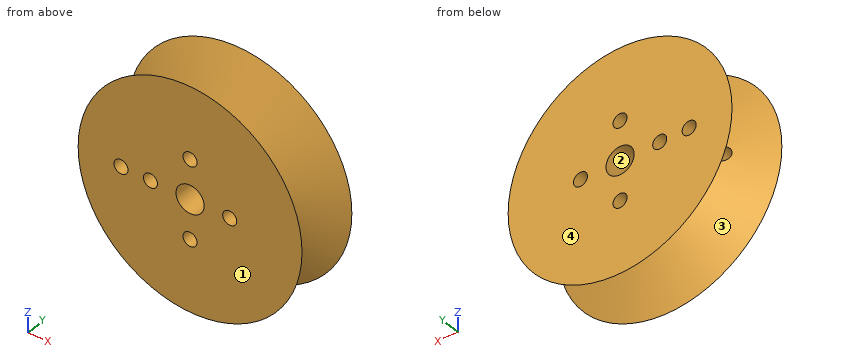
Autodesk Inventor part; units mm, degrees
ref_plane "YZ Plane" through (0, 0, 0) normal (1, 0, 0) x (0, 1, 0)
ref_plane "XZ Plane" through (0, 0, 0) normal (0, 1, 0) x (-1, 0, 0)
ref_plane "XY Plane" through (0, 0, 0) normal (0, 0, 1) x (1, 0, 0)
sketch "Sketch1" plane through (0, 0, 0) normal (0, 1, 0) x (-1, 0, 0)
  circle A0 centre (0, 0) radius 22.225
  dimension "d0" = 44.45
extrude "Extrusion1" add sketch "Sketch1" along normal blind 6.35
chamfer "Chamfer1" distance 12.7 distance2 6.35 1 edges at (22.225, 6.35, 0) measured on face at (-2.0252, 6.35, -4.4852)
sketch "Sketch2" plane through (0, 6.35, 0) normal (0, 1, 0) x (1, 0, 0)
  circle A0 centre (0, 0) radius 22.225
  dimension "d57" = 44.45
extrude "Extrusion2" add sketch "Sketch2" along normal blind 6.35
chamfer "Chamfer2" distance 12.7 distance2 6.35 1 edges at (-22.225, 6.35, 0) measured on face at (17.7764, 6.35, 1.7729)
sketch "Sketch4" plane through (0, 12.7, 0) normal (0, 1, 0) x (1, 0, 0)
  circle A0 centre (0, 0) radius 2.794
  line L0 (0, 0) -> (-7.874, 0)
  line L1 (-7.874, 0) -> (-13.716, 0)
  line L2 (0, 0) -> (0, 7.874)
  line L3 (0, 0) -> (7.874, 0)
  line L4 (0, 0) -> (0, -7.874)
  circle A1 centre (0, -7.874) radius 1.397
  circle A2 centre (7.874, 0) radius 1.397
  circle A3 centre (0, 7.874) radius 1.397
  circle A4 centre (-7.874, 0) radius 1.397
  circle A5 centre (-13.716, 0) radius 1.397
  dimension "d28" = 5.588
  dimension "d29" = 7.874
  dimension "d30" = 5.842
  dimension "d31" = 7.874
  dimension "d32" = 7.874
  dimension "d33" = 7.874
  dimension "d34" = 2.794
  dimension "d35" = 2.794
  dimension "d36" = 2.794
  dimension "d37" = 2.794
  dimension "d38" = 2.794
extrude "Extrusion3" cut sketch "Sketch4" against normal blind 15.24
sketch "Sketch5" plane through (0, 0, 0) normal (0, -1, 0) x (1, 0, 0)
  circle A0 centre (0, 0) radius 2.794
  circle A1 centre (0, 0) radius 11.1125
  dimension "d58" = 22.225
properties part number "String Little Big Wheel V5"
The listing builds one solid part. Answer for the finished solid, in the listing's coordinates (mm). Face numbers are marked on the shaded views. A direction names the side the tool comes from. Coordinates: 2 decimals unless noted, no trailing zeros. Write each loop counter-clockwise with the first axis right and the second up, starting at its lowest first coordinate (ties: lowest second). Pieces come first, ordered by that corner, then holes. Notation, with made-up numbers: (37.25, -11.75) - (84.25, -11.75) arc R33 ccw to (84.25, 23.25) - close; hole circle Ø6 at (-35.75, 57). An arc over 180 degrees is marked (long way). Return JSON: item names as keys, results as strings.
1. Which of the six approach directions +Z, -Z, +X, -X, +Y, -Y give full straight-line access (tool end or side, diameter ignored) to the marked faces 3 and 4?
Final values:
{"face 3": "none", "face 4": "+Z, -Z, +X, -X, +Y"}
2. The part is cut by section A-A on z = 0. Count the separate pieces of the cut face and the enclosed holes in it, then the cut area to 3 significant figures.
Final values:
{"separate pieces": "6", "enclosed holes": "0", "area": "238 mm^2"}
3. Each of these flat-tipped pins is pushed along its axis until it touches: pin 1 Ø2.5 at (x, z) = (7.874, 0) entering from -Y; pin 2 Ø4.5 at (x, z) = (0, 7.874) entering from -Y; pin 3 Ø6 at (y, z) = (4.5, 9) entering from -X. Where does it stop, or does it pass through?
Final values:
{"pin 1": "through", "pin 2": "y = 0", "pin 3": "x = -17.16"}
4. For a pull along Z with two mould halves and no side action, classify the marked faces 1 and 2 as +Z half, -Z half, draft (parallel to the pull), parting line (faces both ways), or undercut.
Final values:
{"face 1": "draft", "face 2": "undercut"}
5. Consider line 1 along X through (y, z) = (8, 0); line 2 along X through (y, z) = (2, 0); line 3 along Z through (x, y) = (0, 4). Determine where each line is inside the solid, lowest interval first.
Final values:
{"line 1": "-12.32 to -9.27, -6.48 to -2.79, 2.79 to 6.48, 9.27 to 12.83", "line 2": "-18.23 to -15.11, -12.32 to -9.27, -6.48 to -2.79, 2.79 to 6.48, 9.27 to 18.23", "line 3": "-14.23 to -9.27, -6.48 to -2.79, 2.79 to 6.48, 9.27 to 14.23"}
6. The part is cut by section C-C on y = 1. Determine the outline of the cut face in (x, z), then the cut area to 3 significant figures.
Final values:
{"outline": "circle Ø40.45 at (0, 0); hole circle Ø2.79 at (-13.72, 0); hole circle Ø2.79 at (-7.87, 0); hole circle Ø5.59 at (0, 0); hole circle Ø2.79 at (0, -7.87); hole circle Ø2.79 at (0, 7.87); hole circle Ø2.79 at (7.87, 0)", "area": "1,230 mm^2"}
